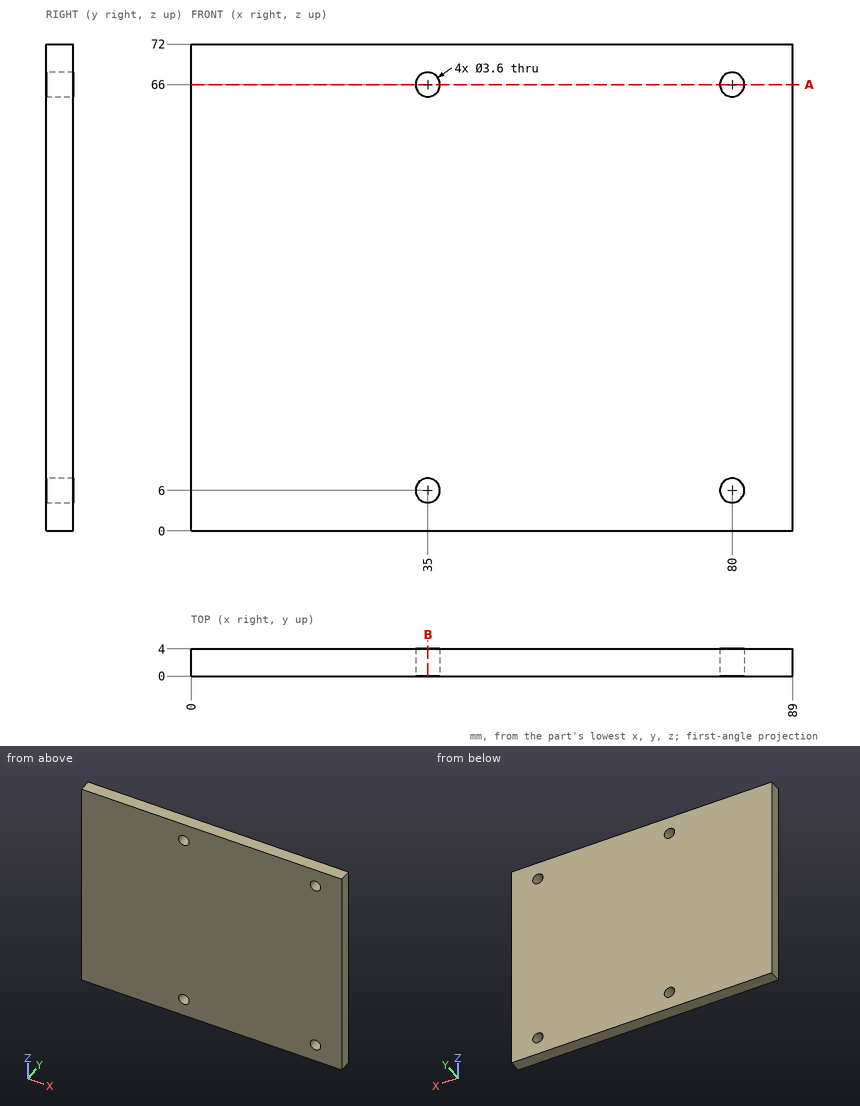
For this review, use the dimensioned drawing (mm, ordinates from the lowest corner) and the shaded views. Coordinates: 2 decimals unless noted, no trailing zeros. Write each loop counter-clockwise with the first axis right and the second up, starting at its lowest first coordinate (ties: lowest second). Pieces come first, ordered by that corner, then holes. Notation, with made-up numbers: (85.25, 53) -> (100.25, 53) arc R20 cw to (100.25, 87) -> close; hole circle Ø5 at (24, 57). An arc over 180 degrees is marked (long way). Put each result on its own line as item: value.
Q1. Take a section at B-B, the plane x = 35. State the section outline as (y, z) points, then the cut area to 3 significant figures.
From the geometry:
outline: (0, 0) -> (4, 0) -> (4, 4.2) -> (0, 4.2) -> close; (0, 7.8) -> (4, 7.8) -> (4, 64.2) -> (0, 64.2) -> close; (0, 67.8) -> (4, 67.8) -> (4, 72) -> (0, 72) -> close
area: 259 mm2
Q2. Wall thickness on L1, parallel to X at y = 2.9, z = 6: over which ranges is the line inside the solid? List them lowest first.
From the geometry:
L1: x = 0 to 33.2, 36.8 to 78.2, 81.8 to 89
Q3. Take a section at A-A, the plane z = 66. State the section outline as (x, y) points, then the cut area to 3 significant figures.
From the geometry:
outline: (0, 0) -> (33.2, 0) -> (33.2, 4) -> (0, 4) -> close; (36.8, 0) -> (78.2, 0) -> (78.2, 4) -> (36.8, 4) -> close; (81.8, 0) -> (89, 0) -> (89, 4) -> (81.8, 4) -> close
area: 327 mm2
